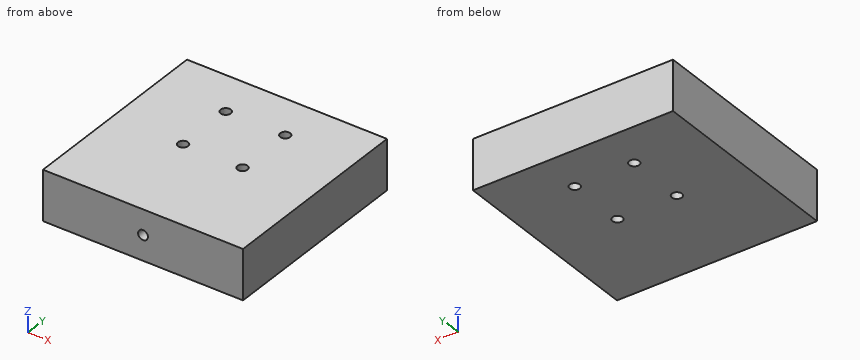
Autodesk Inventor part; units mm, degrees
ref_plane "YZ Plane" through (0, 0, 0) normal (1, 0, 0) x (0, 1, 0)
ref_plane "XZ Plane" through (0, 0, 0) normal (0, 1, 0) x (-1, 0, 0)
ref_plane "XY Plane" through (0, 0, 0) normal (0, 0, 1) x (1, 0, 0)
sketch "Sketch1" plane through (0, 0, 0) normal (0, 0, 1) x (1, 0, 0)
  line L0 (-23.6409, 18.7983) -> (77.9591, 18.7983)
  line L1 (77.9591, 18.7983) -> (77.9591, -82.8017)
  line L2 (77.9591, -82.8017) -> (-23.6409, -82.8017)
  line L3 (-23.6409, -82.8017) -> (-23.6409, 18.7983)
  point P0 (0, 0)
  dimension "d0" = 101.6
  dimension "d1" = 101.6
extrude "Extrusion1" add sketch "Sketch1" along normal blind 25.4
sketch "Sketch2" plane through (0, 0, 25.4) normal (0, 0, 1) x (1, 0, 0)
  line L0 (-23.6409, 18.7983) -> (77.9591, 18.7983)
  line L1 (27.1591, 18.7983) -> (52.8131, 18.7983)
  line L2 (27.1591, 18.7983) -> (1.5051, 18.7983)
  line L3 (1.5051, 18.7983) -> (12.0461, 18.7983)
  line L4 (52.8131, 18.7983) -> (42.2721, 18.7983)
  line L5 (12.0461, 18.7983) -> (12.0461, -3.4267)
  line L6 (12.0461, 18.7983) -> (12.0461, -33.5257)
  line L7 (42.2721, 18.7983) -> (42.2721, -3.4267)
  line L8 (42.2721, -3.4267) -> (42.2721, -33.5257)
  point P0 (0, 0)
  dimension "d4" = 25.654
  dimension "d5" = 25.654
  dimension "d6" = 10.541
  dimension "d7" = 10.541
  dimension "d8" = 22.225
  dimension "d9" = 52.324
hole "Hole1" at (12.0461, -3.4267, 25.4) at (42.2721, -3.4267, 25.4) at (42.2721, -33.5257, 25.4) at (12.0461, -33.5257, 25.4) direction (0, 0, -1) diameter 5.1054 depth 25.4 tip angle 118
sketch "Sketch3" plane through (-23.6409, -82.8017, 0) normal (0, -1, 0) x (1, 0, 0)
  line L0 (101.6, 25.4) -> (0, 25.4)
  line L1 (101.6, 0) -> (0, 0)
  line L2 (50.8, 25.4) -> (50.8, 0)
  line L3 (50.8, 12.7) -> (56.2489, 12.7)
  point P0 (23.6409, 0)
hole "Hole2" at (27.1591, -82.8017, 12.7) direction (0, 1, 0) diameter 4.9784 depth 12.7 tip angle 118
properties part number "mixer mount"
Geometry: final body of the model. Coordinates: model frame, mm. Round coordinates to 2 decimals unless told otherwise and drop trailing zeros. Order: outer loops, then holes, each group sorted by start corner. A loop starts at its lowest first (then second) coordinate and runs counter-clockwise, first axis right, second up. Notation, with made-up numbers: (-29.75, 74.25) -> (-18.75, 74.25) arc R20 cw to (-18.75, 91.25) -> close; hole circle Ø6 at (33.25, 86). An arc over 180 degrees is marked (long way). Use one line per item in the form item = value. Start each with the question number.
1. Cut plane A-A (y = -3.5). Return the cut outline in (x, z), then the cut area to 3 significant figures.
2. Pin query (flat end, axial travel): pin 1 Ø4.5 at (x, y) = (12.05, -3.43) entering from +Z; pin 2 Ø3 at (x, z) = (27.16, 12.7) entering from -Y. Return the tip coordinate at first contact, or that it passes through.
3. Line query: probe 1 along Y at (x, z) = (13, 21.75); probe 2 along X at (y, z) = (-75.5, 12.7); probe 3 along X at (y, z) = (-33, 14). Output: solid intervals per line, ascending.
Solution:
q1.outline = (-23.64, 0) -> (9.49, 0) -> (9.49, 25.4) -> (-23.64, 25.4) -> close; (14.6, 0) -> (39.72, 0) -> (39.72, 25.4) -> (14.6, 25.4) -> close; (44.82, 0) -> (77.96, 0) -> (77.96, 25.4) -> (44.82, 25.4) -> close
q1.area = 2,320 mm^2
q2.pin_1 = through
q2.pin_2 = -69.51
q3.probe_1 = -82.8 to -35.89, -31.16 to -5.79, -1.06 to 18.8
q3.probe_2 = -23.64 to 24.67, 29.65 to 77.96
q3.probe_3 = -23.64 to 9.55, 14.54 to 39.77, 44.77 to 77.96
